Solid Edge part; units mm, degrees
sketch "Sketch1" plane through (0, 0, 0) normal (0, -1, 0) x (1, 0, 0)
  line L0 (-13.5, -5) -> (13.5, -5)
  line L1 (13.5, -5) -> (13.5, 5)
  line L2 (13.5, 5) -> (-13.5, 5)
  line L3 (-13.5, 5) -> (-13.5, -5)
  dimension "D1" = 13.5
  dimension "D2" = 13.5
extrude "Protrusion1" add sketch "Sketch1" along normal mid plane 34.7
sketch "Sketch2" plane through (13.5, 0, 0) normal (1, 0, 0) x (0, 1, 0)
  line L0 (-17.35, 5) -> (-10.85, 5)
  line L1 (-10.85, 5) -> (-10.85, 4.5)
  line L2 (-10.85, 4.5) -> (-17.35, 4.5)
  line L3 (-17.35, 4.5) -> (-17.35, 5)
  dimension "D1" = 17.35
extrude "Cutout1" cut sketch "Sketch2" against normal through all
mirror "Mirror1" about plane through (0, 0, 0) normal (0, -1, 0) of "Cutout1"
sketch "Sketch3" plane through (0, -17.35, -0.25) normal (0, -1, 0) x (1, 0, 0)
  line L0 (0, -4.75) -> (-6, -4.75)
  line L1 (-6, -4.75) -> (-6, 0.25)
  line L2 (-6, 0.25) -> (0, 0.25)
  line L3 (0, 0.25) -> (0, -4.75)
  dimension "D1" = 6
extrude "Cutout3" cut sketch "Sketch3" against normal through all
mirror "Mirror2" about plane through (0, 0, 0) normal (-1, 0, 0) of "Cutout3"
sketch "Sketch4" plane through (0, 0, 5) normal (0, 0, 1) x (0, 1, 0)
  circle A0 centre (-7.5, 10) radius 1.5
  circle A1 centre (7.5, 10) radius 1.5
  circle A2 centre (7.5, -10) radius 1.5
  circle A3 centre (-7.5, -10) radius 1.5
  dimension "D1" = 7.5
  dimension "D2" = 7.5
extrude "ExtrudedCutout_5" cut sketch "Sketch4" against normal blind 3.5
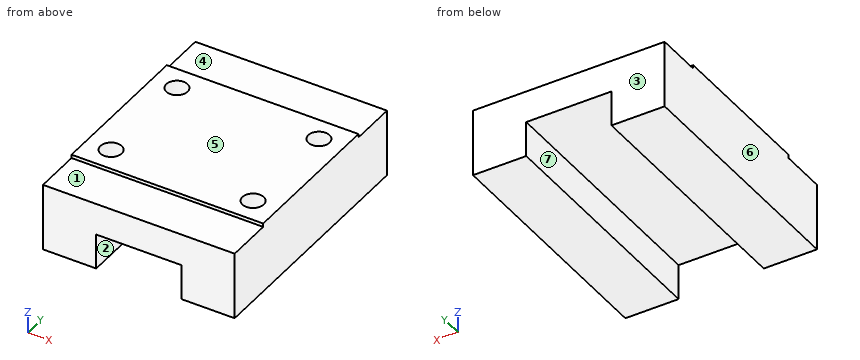
Check sheet for the modelled part. Datum: model origin and axes. Units: mm. Face numbers are marked on the shaded views. A direction names the side the tool comes from. Round coordinates to 2 decimals unless told otherwise and drop trailing zeros. Write each loop counter-clockwise with the first axis right and the second up, starting at its lowest first coordinate (ties: lowest second). Pieces come first, ordered by that corner, then holes. Notation, with made-up numbers: (4, 2) -> (44, 2) arc R18 ccw to (44, 16) -> close; hole circle Ø10 at (17.5, -35). An arc over 180 degrees is marked (long way). One line per question, with ' | ' between items. Start each with the question number.
1. Sectioned sample at D-D, the plane z = 4. Record the cut outline in (x, y).
2. Scan lines: line 1 along Y through (x, z) = (10, 3.95); line 2 along X through (y, z) = (-7.5, 2.6); line 3 along X through (y, z) = (16, -1.75). Record each from-to range of solid material in increasing order. Write a range as from..to.
3. Depth check by flat-ended pin: pin 1 (0.9 mm diameter, centred on x = 10, y = -8, fed in from +Z); pin 2 (5 mm diameter, centred on x = 3.5, y = -14, fed in from +Z); pin 3 (6 mm diameter, centred on x = -1.5, y = 3, fed in from -Z); pin 4 (5 mm diameter, centred on x = 0.5, y = 13, fed in from +Z). Enter the tip coordinate at first touch or a pass-through.
4. Sectioned sample at C-C, the plane y = 2. Record the cut outline in (x, z), then the cut area to 3 significant figures.
5. Sectioned sample at A-A, the plane z = -1. Record the cut outline in (x, y).
6. Release check for a two-part mould opening along X. For the marked faces 5, 6 and 7 record: +X half, -X half, draft (parallel to the pull), parting line (faces both ways), or undercut.
7. Set-up check for the marked faces 1, 2, 3 and 4: record each of +Z, -Z, +X, -X, +Y, -Y from which the full face is reachable in a straight line by a thin tool's end or side.
8. Sectioned sample at B-B, the plane x = 10. Record the cut outline in (y, z).
Taken from the geometry:
1) outline: (-13.5, -17.35) -> (13.5, -17.35) -> (13.5, 17.35) -> (-13.5, 17.35) -> close; hole circle Ø3 at (-10, -7.5); hole circle Ø3 at (-10, 7.5); hole circle Ø3 at (10, -7.5); hole circle Ø3 at (10, 7.5)
2) line 1: y = -17.35..-9, -6..6, 9..17.35 | line 2: x = -13.5..-11.5, -8.5..8.5, 11.5..13.5 | line 3: x = -13.5..-6, 6..13.5
3) pin 1: stops at z = 1.5 | pin 2: stops at z = 4.5 | pin 3: stops at z = 0 | pin 4: stops at z = 5
4) outline: (-13.5, -5) -> (-6, -5) -> (-6, 0) -> (6, 0) -> (6, -5) -> (13.5, -5) -> (13.5, 5) -> (-13.5, 5) -> close | area: 210 mm^2
5) outline: (-13.5, -17.35) -> (-6, -17.35) -> (-6, 17.35) -> (-13.5, 17.35) -> close; (6, -17.35) -> (13.5, -17.35) -> (13.5, 17.35) -> (6, 17.35) -> close
6) face 5: draft | face 6: -X half | face 7: undercut
7) face 1: +Z, +X, -X, -Y | face 2: -Z, +Y, -Y | face 3: +Z, -Z, +X, -X, +Y | face 4: +Z, +X, -X, +Y
8) outline: (-17.35, -5) -> (17.35, -5) -> (17.35, 4.5) -> (10.85, 4.5) -> (10.85, 5) -> (9, 5) -> (9, 1.5) -> (6, 1.5) -> (6, 5) -> (-6, 5) -> (-6, 1.5) -> (-9, 1.5) -> (-9, 5) -> (-10.85, 5) -> (-10.85, 4.5) -> (-17.35, 4.5) -> close
